Verification items for this drawing (mm, ordinates from the low corner). A direction names the side the tool comes from. Give positions to 0.01 mm unless a question says otherwise; leave off trailing zeros. Order: outer loops, then holes, each group sorted by start corner. A loop starts at its lowest first (then second) coordinate and runs counter-clockwise, first axis right, second up.
(1) Gauge pin test, flat ends, axial feed: pin 1 (1 mm diameter, centred on x = 12, y = 2, fed in from +Z); pin 2 (1.5 mm diameter, centred on x = 26.5, y = 1, fed in from -Z); pin 3 (0.9 mm diameter, centred on x = 1.5, y = 1.5, fed in from +Z). Record the tip position at first contact, or that the pin passes through.
(2) Sectioned sample at C-C on x = 4. Record the cut outline in (y, z).
(3) Access from +Z, -Z, +X, -X, +Y, -Y to the whole of each face (thin tool, end or side, straight path). Record for the marked faces 1, 2 and 3.
(4) Sectioned sample at B-B on z = 20.5. Record the cut outline in (x, y), plus the area to 3 significant figures.
(5) Sectioned sample at A-A on y = 1.4. Record the cut outline in (x, z).
(6) Scan lines: L1, parallel to Z at x = 11.75, y = 2.4 (3 decimals); L2, parallel to X at y = 1.2, z = 28; L3, parallel to X at y = 1.6, z = 12.5. Record each from-to range of solid material in increasing order.
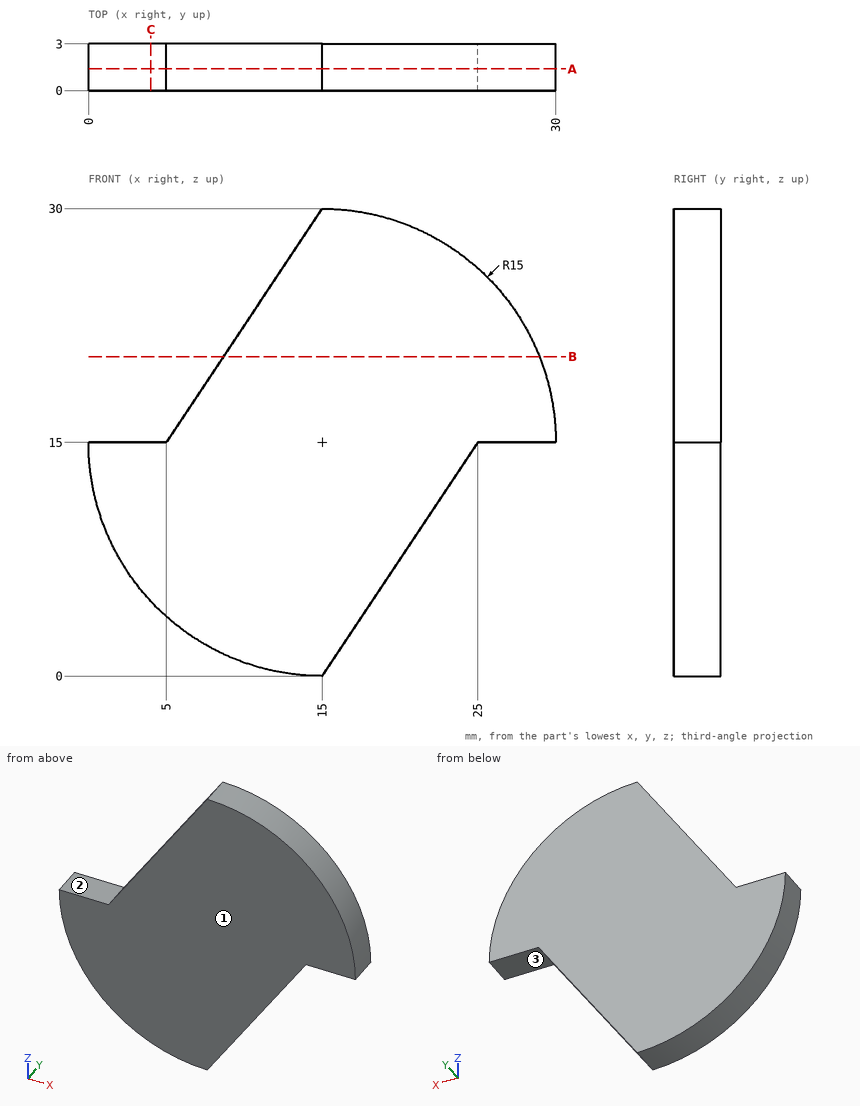
Ans:
1. pin 1: stops at z = 26.25
1. pin 2: stops at z = 15
1. pin 3: stops at z = 15
2. outline: (0, 4.8) - (3, 4.8) - (3, 15) - (0, 15) - close
3. face 1: +Z, -Z, +X, -X, -Y
3. face 2: +Z, -X, +Y, -Y
3. face 3: -Z, +X, +Y, -Y
4. outline: (8.67, 0) - (28.96, 0) - (28.96, 3) - (8.67, 3) - close
4. area: 60.9 mm2
5. outline: (0, 15) arc R15 ccw to (15, 0) - (25, 15) - (30, 15) arc R15 ccw to (15, 30) - (5, 15) - close
6. L1: z = 0.356 to 25.125
6. L2: x = 13.67 to 22.48
6. L3: x = 0.21 to 23.33
